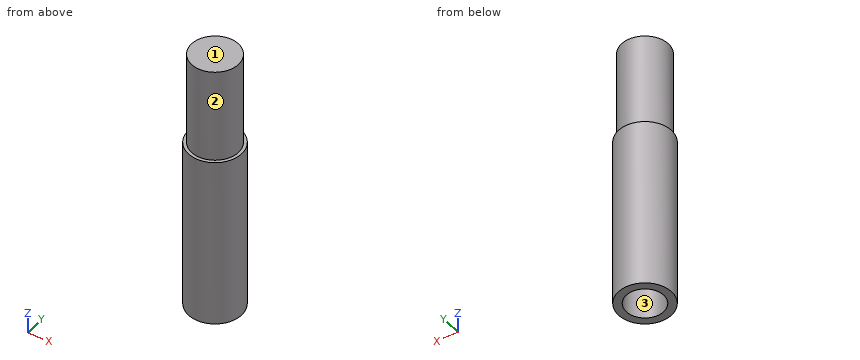
from build123d import *

# Parameters (mm, degrees)
SKETCH1_R           = 7.5
BOSS_EXTRUDE1_DEPTH = 30
SKETCH2_R           = 8.5
SKETCH2_R_2         = 6
BOSS_EXTRUDE2_DEPTH = 55
SKETCH3_R           = 6
BOSS_EXTRUDE3_DEPTH = 3


with BuildPart() as part:
    # Sketch1 → Boss-Extrude1 (new body)
    with BuildSketch(Plane.XY):
        Circle(SKETCH1_R)
    extrude(amount=BOSS_EXTRUDE1_DEPTH)

    # Sketch2 → Boss-Extrude2 (add)
    with BuildSketch(Plane(origin=(0, 0, 0), x_dir=(-1, 0, 0), z_dir=(0, 0, -1))):
        Circle(SKETCH2_R)
        Circle(SKETCH2_R_2, mode=Mode.SUBTRACT)
    extrude(amount=BOSS_EXTRUDE2_DEPTH)

    # Sketch3 → Boss-Extrude3 (add)
    with BuildSketch(Plane(origin=(0, 0, 0), x_dir=(-1, 0, 0), z_dir=(0, 0, -1))):
        Circle(SKETCH3_R)
    extrude(amount=BOSS_EXTRUDE3_DEPTH)


solid = part.part
Model file for the job. Use its own axes, mm. Face numbers are marked on the shaded views. Give positions to 0.01 mm unless a question says otherwise; leave off trailing zeros. Loops run counter-clockwise (first coordinate to the right, second up) from the corner with the lowest first, then second, coordinate; pieces in that order, holes last. Notation, with made-up numbers: (19, 79.5) -> (50, 79.5) arc R25 cw to (50, 106.5) -> close; hole circle Ø6 at (5, 20). An arc over 180 degrees is marked (long way). Use a Markdown table: item, result. Add a question column.
(1) Drop flat-ended pins along their axis: pin 1 Ø1 at (x, y) = (-3.5, -3) entering from -Z; pin 2 Ø1.5 at (y, z) = (6.5, 7) entering from -X; pin 3 Ø2 at (x, z) = (4.5, -2) entering from +Y. Give the stop position or say it passes through.
(2) Slice it at A-A on y = 0. List the corners of the cut face in (x, z), and give its area (3 significant figures).
(3) Slice it at C-C on z = -16.5. List the corners of the cut face in (x, y).
(4) Slice it at D-D on y = -6.75. List the corners of the cut face in (x, z), and give its area (3 significant figures).
(5) Wall check: line 1 along Y through (x, z) = (0, -30.5); line 2 along Z through (x, y) = (6, -5.25); line 3 along Y through (x, z) = (1, -8). Give the ranges that are in metal, low to high.
(6) Mould opens along Y. For the marked faces 1, 2 and 3 say: +Y half, -Y half, draft (parallel to the pull), parting line (faces both ways), or undercut.
Filled sheet:
| question | item | result |
|---|---|---|
| 1 | pin 1 | z = -3 |
| 1 | pin 2 | x = -4.82 |
| 1 | pin 3 | y = 7.75 |
| 2 | outline | (-8.5, -55) -> (-6, -55) -> (-6, -3) -> (6, -3) -> (6, -55) -> (8.5, -55) -> (8.5, 0) -> (7.5, 0) -> (7.5, 30) -> (-7.5, 30) -> (-7.5, 0) -> (-8.5, 0) -> close |
| 2 | area | 761 mm2 |
| 3 | outline | circle Ø17 at (0, 0); hole circle Ø12 at (0, 0) |
| 4 | outline | (-5.17, -55) -> (5.17, -55) -> (5.17, 0) -> (3.27, 0) -> (3.27, 30) -> (-3.27, 30) -> (-3.27, 0) -> (-5.17, 0) -> close |
| 4 | area | 764 mm2 |
| 5 | line 1 | -8.5 to -6, 6 to 8.5 |
| 5 | line 2 | -55 to 0 |
| 5 | line 3 | -8.44 to -5.92, 5.92 to 8.44 |
| 6 | face 1 | draft |
| 6 | face 2 | parting line |
| 6 | face 3 | undercut |
